from build123d import *

# Parameters (mm, degrees)
F1_DEPTH  = 125
F2_R      = 1.85
F3_DEPTH  = 4
F5_DEPTH  = 3
F7_R      = 6
F8_DEPTH  = 25
F10_R     = 6
F11_DEPTH = 25


with BuildPart() as f1:
    # F0 (on Front) → F1 (new body)
    with BuildSketch(Plane.XZ):
        Polygon((27.424138, 47.5), (-27.424138, 47.5), (-23.960036, 41.5), (23.960036, 41.5), align=None)
    extrude(amount=F1_DEPTH)

    # F2 (on face) → F3 (cut)
    with BuildSketch(Plane(origin=(0, 0, 41.5), x_dir=(1, 0, 0), z_dir=(0, 0, -1))):
        with BuildLine():
            ThreePointArc((-13.830018, 120), (-11.980018, 118.15), (-10.130018, 120))
            Line((-10.130018, 120), (-13.830018, 120))
        make_face()
        with BuildLine():
            Line((-13.830018, 120), (-10.130018, 120))
            ThreePointArc((-10.130018, 120), (-11.980018, 121.85), (-13.830018, 120))
        make_face()
        with Locations((11.980018, 120)):
            Circle(F2_R)
        with BuildLine():
            ThreePointArc((-13.830018, 23), (-11.980018, 21.15), (-10.130018, 23))
            Line((-10.130018, 23), (-13.830018, 23))
        make_face()
        with BuildLine():
            Line((-13.830018, 23), (-10.130018, 23))
            ThreePointArc((-10.130018, 23), (-11.980018, 24.85), (-13.830018, 23))
        make_face()
        with Locations((11.980018, 23)):
            Circle(F2_R)
    extrude(amount=-F3_DEPTH, mode=Mode.SUBTRACT)

    # F4 (on face) → F5 (join)
    with BuildSketch(Plane.XY.offset(47.5)):
        with BuildLine():
            ThreePointArc((4.419879, -61.002997), (6.484743, -58.434913), (7.172588, -55.212246))
            ThreePointArc((7.172588, -55.212246), (0.243912, -49.679184), (-6.684764, -55.212246))
            ThreePointArc((-6.684764, -55.212246), (-7.10843, -58.494572), (-6.503523, -61.748377))
            ThreePointArc((-6.503523, -61.748377), (-4.034953, -66.068801), (0.243912, -68.608727))
            ThreePointArc((0.243912, -68.608727), (1.663957, -64.439127), (4.419879, -61.002997))
        make_face()
    extrude(amount=F5_DEPTH)

    # F7 (on face) → F8 (cut)
    with BuildSketch(Plane(origin=(-23.960036, 0, 41.5), x_dir=(0.866025, 0, 0.5), z_dir=(0.5, 0, -0.866025))):
        with Locations((0, 62.5)):
            Circle(F7_R)
    extrude(amount=F8_DEPTH, mode=Mode.SUBTRACT)

    # F10 (on face) → F11 (cut)
    with BuildSketch(Plane(origin=(23.960036, 0, 41.5), x_dir=(0.866025, 0, -0.5), z_dir=(0.5, 0, 0.866025))):
        with Locations((0, -62.5)):
            Circle(F10_R)
    extrude(amount=-F11_DEPTH, mode=Mode.SUBTRACT)


solid = f1.part
Work out the finished part from the listing and answer in its coordinate system (mm). A direction names the side the tool comes from. Coordinates: 2 decimals unless noted, no trailing zeros. Order: outer loops, then holes, each group sorted by start corner. A loop starts at its lowest first (then second) coordinate and runs counter-clockwise, first axis right, second up. Notation, with made-up numbers: (49.25, 62) - (73.25, 62) arc R11 ccw to (73.25, 68) - close; hole circle Ø4 at (80, 45). An arc over 180 degrees is marked (long way). Put each result on its own line as item: value. Start each with the question number.
1) Find section D-D (y = -64). Give the vertices of the cut face in (x, z).
2) Find section A-A (y = -120). Give the vertices of the cut face in (x, z), plus the area to 3 significant figures.
3) Find section B-B (x = 2.5). Give the vertices of the cut face in (y, z).
4) Flat-ended cylindrical pins translate along their axes: pin 1 (3.5 mm diameter, centred on x = 11.98, y = -120, fed in from -Z); pin 2 (1 mm diameter, centred on x = -5.5, y = -66.5, fed in from +Z); pin 3 (1.5 mm diameter, centred on x = -13.5, z = 49, fed in from +Y). Find the tip coordinate at first contact, or state that the pin passes through.
5) For faces 4 (the cylindrical face through (18.1, -62.37, 43.35)), 5 (the cylindrical face through (-4.1, -66, 49)), 6 (the flat face through (0, -62, 41.5)), determine the directions among +Z, -Z, +X, -X, +Y, -Y from which every point of the face is accessible in a straight line to the end or side of a thin tool.
6) Find section C-C (z = 43.25). State how many separate pieces and enclosed holes the cut face has, plus the area to 3 significant figures.
7) Find the intervals of material crossed by line 1 (X direction, y = -23, z = 42.95); line 2 (Y direction, x = -13, z = 45.25); line 3 (Z direction, x = 9, y = -47), in increasing order. Write a range as from..to.
8) For a pull along X with two mould halves and no side action, classify faces 1 (the flat face through (12, -23, 45.5)), 2 (the cylindrical face through (-7.11, -58.45, 48.98)), 3 (the cylindrical face through (6.465, -58.477, 48.979)) as released by +X, released by -X, zero draft, split by the parting line, or undercut.
Results list:
1. outline: (-27.42, 47.5) - (-23.96, 41.5) - (-18.93, 44.4) - (-17.25, 41.5) - (17.25, 41.5) - (18.93, 44.4) - (23.96, 41.5) - (27.42, 47.5) - (1.92, 47.5) - (1.92, 50.5) - (-5.59, 50.5) - (-5.59, 47.5) - close
2. outline: (-27.42, 47.5) - (-23.96, 41.5) - (-13.83, 41.5) - (-13.83, 45.5) - (-10.13, 45.5) - (-10.13, 41.5) - (10.13, 41.5) - (10.13, 45.5) - (13.83, 45.5) - (13.83, 41.5) - (23.96, 41.5) - (27.42, 47.5) - close
2. area: 279 mm^2
3. outline: (-125, 41.5) - (0, 41.5) - (0, 47.5) - (-50.05, 47.5) - (-50.05, 50.5) - (-63.12, 50.5) - (-63.12, 47.5) - (-125, 47.5) - close
4. pin 1: stops at z = 45.5
4. pin 2: stops at z = 47.5
4. pin 3: passes through
5. face 4: -Z
5. face 5: +Z, -X, -Y
5. face 6: -Z, +X, -X, +Y, -Y
6. separate pieces: 1
6. enclosed holes: 6
6. area: 6,160 mm^2
7. line 1: x = -24.8..-13.83, -10.13..10.13, 13.83..24.8
7. line 2: y = -125..-121.54, -118.46..-24.54, -21.46..0
7. line 3: z = 41.5..47.5
8. face 1: undercut
8. face 2: released by -X
8. face 3: released by +X
